Geometry: final body of the model. Coordinates: model frame, mm. Face numbers are marked on the shaded views. A direction names the side the tool comes from. Round coordinates to 2 decimals unless told otherwise and drop trailing zeros. Loops run counter-clockwise (first coordinate to the right, second up) from the corner with the lowest first, then second, coordinate; pieces in that order, holes last. Notation, with made-up numbers: (66.5, -32.75) - (102.5, -32.75) arc R23 cw to (102.5, -14.75) - close; hole circle Ø10 at (47.5, 27). An arc over 180 degrees is marked (long way). Answer as CSV lines item,"result".
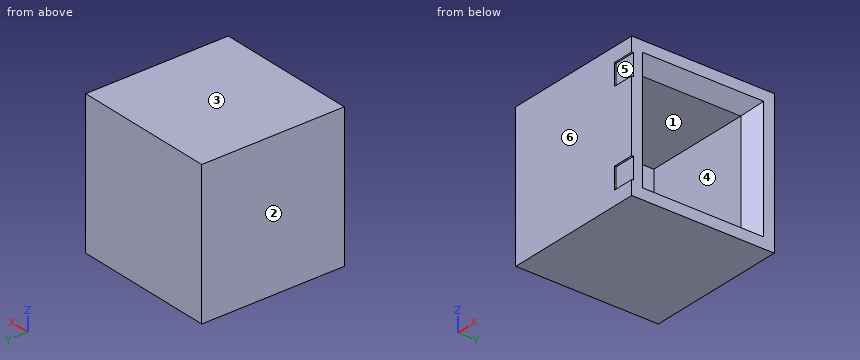
from build123d import *

# Parameters (mm, degrees)
F0_W     = 200
F0_H     = 200
F1_DEPTH = 200
F2_W     = 170
F2_H     = 170
F3_DEPTH = 25
F3_TAPER = 25
F4_W     = 146.6846170923
F4_H     = 146.6846170923
F5_DEPTH = 150
F6_W     = 30
F6_H     = 30
F7_DEPTH = 2.5


with BuildPart() as f1:
    # F0 (on Top) → F1 (new body)
    with BuildSketch(Plane.XY):
        with Locations((100, 100)):
            Rectangle(F0_W, F0_H)
    extrude(amount=F1_DEPTH)

    # F2 (on face) → F3 (cut)
    with BuildSketch(Plane.YZ.offset(200)):
        with Locations((100, 100)):
            Rectangle(F2_W, F2_H)
    extrude(amount=-F3_DEPTH, taper=F3_TAPER, mode=Mode.SUBTRACT)

    # F4 (on face) → F5 (cut)
    with BuildSketch(Plane.YZ.offset(175)):
        with Locations((100, 100)):
            Rectangle(F4_W, F4_H)
    extrude(amount=-F5_DEPTH, mode=Mode.SUBTRACT)

    # F6 (on face) → F7 (cut)
    with BuildSketch(Plane.XZ):
        with Locations((185, 165)):
            Rectangle(F6_W, F6_H)
        with Locations((185, 35)):
            Rectangle(F6_W, F6_H)
    extrude(amount=-F7_DEPTH, mode=Mode.SUBTRACT)


solid = f1.part
(1) Draft query along Z for the marked faces 1, 2 and 3. Return one class per face: pulls with the +Z half, pulls with the -Z half, needs draft (parallel to the pull), parting line crosses it, or undercut.
Findings below:
face 1,"undercut"
face 2,"needs draft"
face 3,"pulls with the +Z half"
(2) Section A-A (x = 118.5). Output: boundary loops of the cut face in (y, z), and give its area (3 significant figures).
Findings below:
outline,"(0, 0) - (200, 0) - (200, 200) - (0, 200) - close; hole (26.66, 26.66) - (173.34, 26.66) - (173.34, 173.34) - (26.66, 173.34) - close"
area,"18,500 mm2"
(3) Material intervals for line 1 along Y through (x, z) = (147.5, 104.5); line 2 along X through (y, z) = (127, 122), sorted ascending.
Findings below:
line 1,"0 to 26.66, 173.34 to 200"
line 2,"0 to 25"
(4) Access query for the marked faces 4, 5 and 6. Directions: +Z, -Z, +X, -X, +Y, -Y. A direction counts if a zero-diameter tool reaches every point of the face in a straight line with its end or side. Return the directions, or none.
Findings below:
face 4,"+X"
face 5,"+X, -Y"
face 6,"+Z, -Z, +X, -X, -Y"
(5) Pin query (flat end, axial travel): P1, Ø2, axis at x = 181.5, y = 1.5, coming from the -Z side; P2, Ø15, axis at x = 179, z = 158, coming from the -Y side; P3, Ø8, axis at y = 23, z = 140, coming from the +X side; P4, Ø3, axis at y = 0.5, z = 163.5, coming from the +X side. Return the tip coordinate at first contact, or that it passes through.
Findings below:
P1,"z = 0"
P2,"y = 2.5"
P3,"x = 191.42"
P4,"x = 170"
